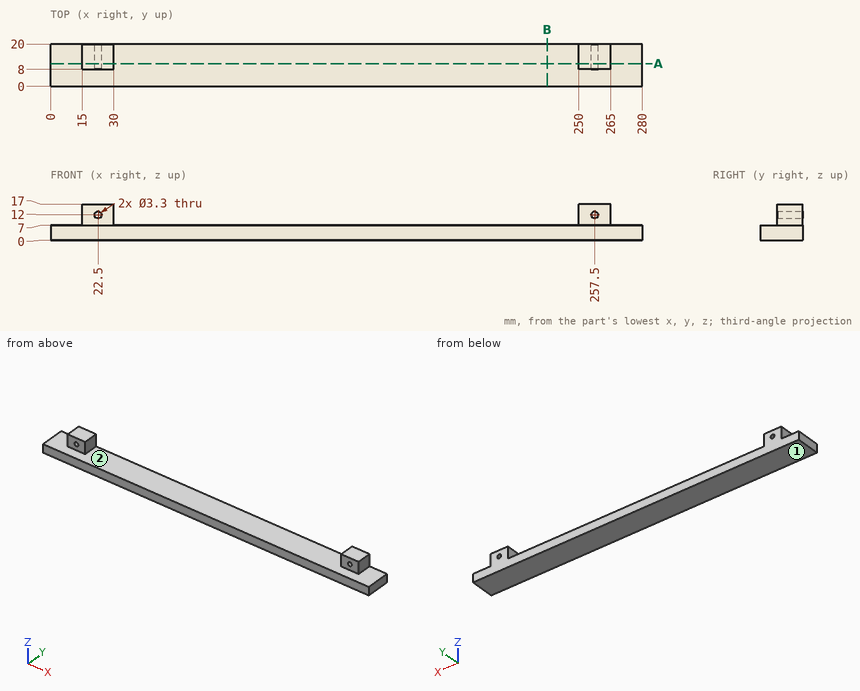
Input: dimensioned drawing with shaded views. Units: mm. Origin: part minimum x, y, z. Give positions to 0.01 mm unless a question says otherwise; leave off trailing zeros. Write each loop counter-clockwise with the first axis right and the second up, starting at its lowest first coordinate (ties: lowest second). Pieces come first, ordered by that corner, then holes. Notation, with made-up numbers: (41, 26) -> (51, 26) arc R13 cw to (51, 35) -> close; hole circle Ø8 at (57.25, 12.5). An arc over 180 degrees is marked (long way). Answer as a JSON object with one key per item and string values.
1. Ray query, probe 1 along X at (y, z) = (10.5, 12); probe 2 along Z at (x, y) = (257.5, 12.75); probe 3 along X at (y, z) = (9.25, 7.75). Return the intervals inside material, ascending. Write a range as from..to.
Ans:
{"probe 1": "x = 15..20.85, 24.15..30, 250..255.85, 259.15..265", "probe 2": "z = 0..10.35, 13.65..17", "probe 3": "x = 15..30, 250..265"}
2. Mould query, pull axis X, two halves, no side actions, for the marked faces 1 and 2. Classes: pulls with the +X half, pulls with the -X half, needs draft (parallel to the pull), parting line crosses it, or undercut.
Ans:
{"face 1": "needs draft", "face 2": "undercut"}
3. Cut plane A-A on y = 10.75. Output: boundary loops of the cut face in (x, z), and give its area (3 significant figures).
Ans:
{"outline": "(0, 0) -> (280, 0) -> (280, 7) -> (265, 7) -> (265, 17) -> (250, 17) -> (250, 7) -> (30, 7) -> (30, 17) -> (15, 17) -> (15, 7) -> (0, 7) -> close; hole circle Ø3.3 at (22.5, 12); hole circle Ø3.3 at (257.5, 12)", "area": "2,240 mm^2"}
4. Contact query for flat-ended pins moving along their axis: pin 1 (10 mm diameter, centred on x = 136, y = 4.5, fed in from +Z); pin 2 (8 mm diameter, centred on x = 21.5, z = 11.5, fed in from -Y); pin 3 (5 mm diameter, centred on x = 134.5, z = 10, fed in from -Y). Output: stop coordinate, or through.
Ans:
{"pin 1": "stops at z = 7", "pin 2": "stops at y = 8", "pin 3": "passes through"}
5. Cut plane B-B on x = 235. Output: boundary loops of the cut face in (y, z).
Ans:
{"outline": "(0, 0) -> (20, 0) -> (20, 7) -> (0, 7) -> close"}
